from build123d import *

# Parameters (mm, degrees)
SKETCH1_W                      = 146.142719433
SKETCH1_H                      = 29.841975708
BOSS_EXTRUDE1_DEPTH            = 4
SKETCH2_W                      = 42.4
SKETCH2_H                      = 21
CUT_EXTRUDE1_DEPTH             = 120.920808812
SKETCH3_W                      = 42.4
SKETCH3_H                      = 21
CUT_EXTRUDE2_DEPTH             = 120.920808812
BOSS_EXTRUDE2_DEPTH            = 25
BOSS_EXTRUDE3_DEPTH            = 25
BOSS_EXTRUDE4_DEPTH            = 25
BOSS_EXTRUDE5_DEPTH            = 25
BOSS_EXTRUDE6_DEPTH            = 25
BOSS_EXTRUDE7_DEPTH            = 25
F_3_1_3_1_DIAMETER_HOLE1_D     = 3.1
F_3_1_3_1_DIAMETER_HOLE1_DEPTH = 29
F_3_1_3_1_DIAMETER_HOLE2_D     = 3.1
FILLET1_R                      = 1
FILLET2_R                      = 2
FILLET3_R                      = 8


with BuildPart() as part:
    # Sketch1 → Boss-Extrude1 (new body)
    with BuildSketch(Plane.XY.offset(29.720987506)):
        with Locations((40.928641953, 22.079012221)):
            Rectangle(SKETCH1_W, SKETCH1_H)
    extrude(amount=-BOSS_EXTRUDE1_DEPTH)

    # Sketch2 → Cut-Extrude1 (cut, through all)
    with BuildSketch(Plane.XY.offset(29.720987506)):
        with Locations((0, 22.079011948)):
            Rectangle(SKETCH2_W, SKETCH2_H)
    extrude(amount=-CUT_EXTRUDE1_DEPTH, mode=Mode.SUBTRACT)

    # Sketch3 → Cut-Extrude2 (cut, through all)
    with BuildSketch(Plane(origin=(0, 0, 25.720987506), x_dir=(-1, 0, 0), z_dir=(0, 0, -1))):
        with Locations((-81.857283905, 22.079012494)):
            Rectangle(SKETCH3_W, SKETCH3_H)
    extrude(amount=-CUT_EXTRUDE2_DEPTH, mode=Mode.SUBTRACT)

    # Sketch4 → Boss-Extrude2 (add)
    with BuildSketch(Plane(origin=(0, 0, 25.720987506), x_dir=(-1, 0, 0), z_dir=(0, 0, -1))):
        with BuildLine():
            Line((28.579999925, 27.164011892), (28.579999925, 24.579012633))
            Line((28.579999925, 24.579012633), (25.700002555, 24.579012633))
            ThreePointArc((25.700002555, 24.579012633), (25.204684679, 24.573625897), (24.72588263, 24.446671519))
            ThreePointArc((24.72588263, 24.446671519), (22.771679916, 24.362550773), (21.2, 25.52694194))
            Line((21.2, 25.52694194), (21.2, 31.476505426))
            ThreePointArc((21.2, 31.476505426), (26.12739861, 31.437827499), (28.579999925, 27.164011892))
        make_face()
    extrude(amount=BOSS_EXTRUDE2_DEPTH)

    # Sketch5 → Boss-Extrude3 (add)
    with BuildSketch(Plane(origin=(0, 0, 25.720987506), x_dir=(-1, 0, 0), z_dir=(0, 0, -1))):
        with BuildLine():
            Line((25.700002576, 19.579012066), (28.580000075, 19.579012066))
            Line((28.580000075, 19.579012066), (28.580000075, 16.994011892))
            ThreePointArc((28.580000075, 16.994011892), (26.127398683, 12.720196248), (21.2, 12.68151847))
            Line((21.2, 12.68151847), (21.2, 18.631083048))
            ThreePointArc((21.2, 18.631083048), (22.771680162, 19.795473883), (24.725882875, 19.711353108))
            ThreePointArc((24.725882875, 19.711353108), (25.204684818, 19.58439879), (25.700002576, 19.579012066))
        make_face()
    extrude(amount=BOSS_EXTRUDE3_DEPTH)

    # Sketch6 → Boss-Extrude4 (add)
    with BuildSketch(Plane(origin=(0, 0, 25.720987506), x_dir=(-1, 0, 0), z_dir=(0, 0, -1))):
        with BuildLine():
            Line((-107.557286435, 24.579012773), (-110.437283905, 24.579012773))
            Line((-110.437283905, 24.579012773), (-110.437283905, 27.164012494))
            ThreePointArc((-110.437283905, 27.164012494), (-107.984682551, 31.43782812), (-103.057283905, 31.476505972))
            Line((-103.057283905, 31.476505972), (-103.057283905, 25.52694194))
            ThreePointArc((-103.057283905, 25.52694194), (-104.628963944, 24.362550939), (-106.583166657, 24.4466717))
            ThreePointArc((-106.583166657, 24.4466717), (-107.061968635, 24.573626043), (-107.557286435, 24.579012773))
        make_face()
    extrude(amount=BOSS_EXTRUDE4_DEPTH)

    # Sketch7 → Boss-Extrude5 (add)
    with BuildSketch(Plane(origin=(0, 0, 25.720987506), x_dir=(-1, 0, 0), z_dir=(0, 0, -1))):
        with BuildLine():
            Line((-110.437283905, 16.994012494), (-110.437283905, 19.579012206))
            Line((-110.437283905, 19.579012206), (-107.557286506, 19.579012206))
            ThreePointArc((-107.557286506, 19.579012206), (-107.06196867, 19.584398936), (-106.583166657, 19.711353289))
            ThreePointArc((-106.583166657, 19.711353289), (-104.628963944, 19.795474049), (-103.057283905, 18.631083048))
            Line((-103.057283905, 18.631083048), (-103.057283905, 12.681519016))
            ThreePointArc((-103.057283905, 12.681519016), (-107.984682551, 12.720196869), (-110.437283905, 16.994012494))
        make_face()
    extrude(amount=BOSS_EXTRUDE5_DEPTH)

    # Sketch8 → Boss-Extrude6 (add)
    with BuildSketch(Plane(origin=(0, 0, 25.720987506), x_dir=(-1, 0, 0), z_dir=(0, 0, -1))):
        with BuildLine():
            Line((-28.58, 16.994011948), (-28.58, 27.164011948))
            ThreePointArc((-28.58, 27.164011948), (-26.127398647, 31.437827573), (-21.2, 31.476505426))
            Line((-21.2, 31.476505426), (-21.2, 12.68151847))
            ThreePointArc((-21.2, 12.68151847), (-26.127398647, 12.720196322), (-28.58, 16.994011948))
        make_face()
    extrude(amount=BOSS_EXTRUDE6_DEPTH)

    # Sketch9 → Boss-Extrude7 (add)
    with BuildSketch(Plane(origin=(0, 0, 25.720987506), x_dir=(-1, 0, 0), z_dir=(0, 0, -1))):
        with BuildLine():
            Line((-53.277283905, 27.164012494), (-53.277283905, 16.994012494))
            ThreePointArc((-53.277283905, 16.994012494), (-55.729885258, 12.720196869), (-60.657283905, 12.681519016))
            Line((-60.657283905, 12.681519016), (-60.657283905, 31.476505972))
            ThreePointArc((-60.657283905, 31.476505972), (-55.729885258, 31.43782812), (-53.277283905, 27.164012494))
        make_face()
    extrude(amount=BOSS_EXTRUDE7_DEPTH)

    # Ø3.1 (3.1) Diameter Hole1
    with Locations(Plane.XY.offset(29.720987506)):
        with Locations((40.928641952, 15.618518294), (40.928641952, 28.039506364)):
            Hole(F_3_1_3_1_DIAMETER_HOLE1_D / 2, depth=F_3_1_3_1_DIAMETER_HOLE1_DEPTH)

    # Ø3.1 (3.1) Diameter Hole2 (through all)
    with Locations(Plane.XY.offset(29.720987506)):
        with Locations((-23.63, 27.164011948), (-23.63, 16.994011948), (23.63, 16.994011948), (23.63, 27.164011948), (58.227283905, 16.994012494), (58.227283905, 27.164012494), (105.487283905, 16.994012494), (105.487283905, 27.164012494)):
            Hole(F_3_1_3_1_DIAMETER_HOLE2_D / 2)

    # Fillet1
    fillet1_edges = [part.edges().sort_by_distance(p)[0] for p in [
        (103.057283905, 18.631083048, 13.220987506),
        (-21.2, 25.52694194, 13.220987506),
        (-21.2, 18.631083048, 13.220987506),
        (103.057283905, 25.52694194, 13.220987506),
    ]]
    fillet(fillet1_edges, radius=FILLET1_R)

    # Fillet2
    fillet2_edges = [part.edges().sort_by_distance(p)[0] for p in [
        (110.437283905, 19.579012206, 13.220987506),
        (-28.579999925, 24.579012633, 13.220987506),
        (-28.580000075, 19.579012066, 13.220987506),
        (110.437283905, 24.579012773, 13.220987506),
    ]]
    fillet(fillet2_edges, radius=FILLET2_R)

    # Fillet3
    fillet3_edges = [part.edges().sort_by_distance(p)[0] for p in [
        (-32.142717764, 7.158024367, 27.720987506),
        (-32.142717764, 37.000000075, 27.720987506),
        (114.000001669, 37.000000075, 27.720987506),
        (114.000001669, 7.158024367, 27.720987506),
    ]]
    fillet(fillet3_edges, radius=FILLET3_R)


solid = part.part
Geometry check sheet. Reference: the model listing, model coordinates, mm. A direction names the side the tool comes from. Coordinates: 2 decimals unless noted, no trailing zeros. Order: outer loops, then holes, each group sorted by start corner. A loop starts at its lowest first (then second) coordinate and runs counter-clockwise, first axis right, second up. Notation, with made-up numbers: (6, 60) - (60, 60) arc R24 cw to (60, 80) - close; hole circle Ø7 at (-22.5, -31). An arc over 180 degrees is marked (long way). Answer in a Markdown table with one row per item. Add a question column.
1) Release check for a two-part mould opening along X. For faces 1 (the flat face through (40, 7.158, 28)), 2 (the flat face through (0, 11.579, 28)), 3 (the flat face through (-32.143, 22, 28)) record: +X half, -X half, draft (parallel to the pull), parting line (faces both ways), or undercut.
2) Material ranges on line 1 along Y through (x, z) = (-23.63, 18); line 2 along X through (y, z) = (23, 27.75); line 3 along Y through (x, z) = (-4, 26.25), recorded low to high. Write a range as [from, to].
3) Cross-section at A-A, the plane x = 90. Record the cut outline in (y, z).
4) Set-up check for faces 4 (the flat face through (82, 11.579, 28)), 5 (the flat face through (25, 22, 0.721)), 6 (the flat face through (40, 22, 25.721)): record each of +Z, -Z, +X, -X, +Y, -Y from which the full face is reachable in a straight line by a thin tool's end or side.
5) Cross-section at B-B, the plane x = 23.63. Record the cut outline in (y, z).
6) Gauge pin test, flat ends, axial feed: P1, Ø3.5, axis at x = 105.49, y = 16.99, coming from the +Z side; P2, Ø5, axis at y = 24.5, z = 8.5, coming from the -X side; P3, Ø8, axis at x = 63.5, z = 15.5, coming from the -Y side; P4, Ø6.5, axis at y = 17.5, z = 19.5, coming from the +X side. Record the tip position at first contact, or that the pin passes through.
7) Cross-section at D-D, the plane y = 34.75. Record the cut outline in (x, z).
8) Cross-section at C-C, the plane z = 22. State how many separate pieces and enclosed holes the cut face has, then the cut area to 3 significant figures.
Check result:
| question | item | result |
|---|---|---|
| 1 | face 1 | draft |
| 1 | face 2 | undercut |
| 1 | face 3 | -X half |
| 2 | line 1 | y = [12.04, 15.44], [18.54, 19.92], [24.23, 25.61], [28.71, 32.11] |
| 2 | line 2 | x = [-32.14, -21.2], [21.2, 60.66], [103.06, 114] |
| 2 | line 3 | y = [7.16, 11.58], [32.58, 37] |
| 3 | outline | (7.16, 25.72) - (11.58, 25.72) - (11.58, 29.72) - (7.16, 29.72) - close; (32.58, 25.72) - (37, 25.72) - (37, 29.72) - (32.58, 29.72) - close |
| 4 | face 4 | +Z, -Z |
| 4 | face 5 | -Z, +X, -X, +Y, -Y |
| 4 | face 6 | -Z |
| 5 | outline | (7.16, 25.72) - (12.04, 25.72) - (12.04, 0.72) - (15.44, 0.72) - (15.44, 29.72) - (7.16, 29.72) - close; (18.54, 0.72) - (25.61, 0.72) - (25.61, 29.72) - (18.54, 29.72) - close; (28.71, 0.72) - (32.11, 0.72) - (32.11, 25.72) - (37, 25.72) - (37, 29.72) - (28.71, 29.72) - close |
| 6 | P1 | stops at z = 29.72 |
| 6 | P2 | stops at x = -28.58 |
| 6 | P3 | stops at y = 12.21 |
| 6 | P4 | stops at x = 110.44 |
| 7 | outline | (-29.7, 25.72) - (111.56, 25.72) - (111.56, 29.72) - (-29.7, 29.72) - close |
| 8 | separate pieces | 6 |
| 8 | enclosed holes | 8 |
| 8 | area | 410 mm² |
